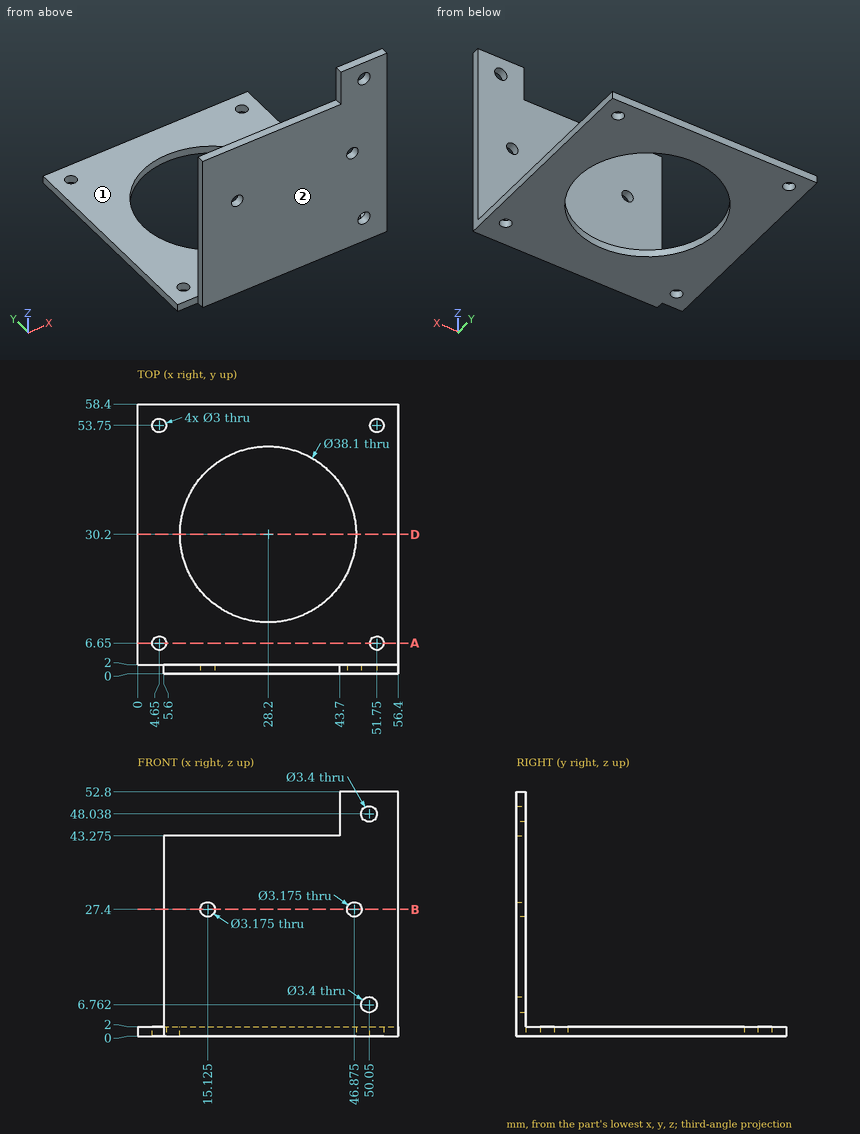
Geometry check sheet. Reference: drawing and pictorial views, mm from the part's lowest x, y, z. A direction names the side the tool comes from. Give positions to 0.01 mm unless a question says otherwise; leave off trailing zeros. Loops run counter-clockwise (first coordinate to the right, second up) from the corner with the lowest first, then second, coordinate; pieces in that order, holes last. Notation, with made-up numbers: M 55,-39.75 L 96,-39.75 A28 ccw 96,-15.75 Z; hole C 17,64 d8. An arc over 180 degrees is marked long. Use a Markdown table: item, result. Add a question column.
Q1. Sectioned sample at A-A, the plane y = 6.65. Record the cut outline in (x, z), then the cut area to 3 significant figures.
Q2. Tool access check on the marked faces 1 and 2. Record the directions out of +Z, -Z, +X, -X, +Y, -Y that give a thin tool (end or side, any length) a straight path to the whole face; none if there is none.
Q3. Scan lines: line 1 along X through (y, z) = (1.3, 27.4); line 2 along Y through (x, z) = (51.75, 0.4); line 3 along X through (y, z) = (30, 1). Record each from-to range of solid material in increasing order. Write a range as [from, to].
Q4. Sectioned sample at D-D, the plane y = 30.2. Record the cut outline in (x, z), then the cut area to 3 significant figures.
Q5. Sectioned sample at B-B, the plane z = 27.4. Record the cut outline in (x, y).
Q6. Go/stop test with flat-tipped pins: pin 1 (1.6 mm diameter, centred on x = 1.5, z = 1, fed in from -Y); pin 2 (1 mm diameter, centred on x = 27.5, y = 1, fed in from +Z) (1 decimal); pin 3 (2 mm diameter, centred on y = 1, z = 13, fed in from -X). Record where each tip stops, or that it passes through.
Verdict:
| question | item | result |
|---|---|---|
| 1 | outline | M 0,0 L 3.15,0 L 3.15,2 L 0,2 Z; M 6.15,0 L 50.25,0 L 50.25,2 L 6.15,2 Z; M 53.25,0 L 56.4,0 L 56.4,2 L 53.25,2 Z |
| 1 | area | 101 mm^2 |
| 2 | face 1 | +Z, +X, -X, +Y |
| 2 | face 2 | +Z, -Z, +X, -X, -Y |
| 3 | line 1 | [5.6, 13.54], [16.71, 45.29], [48.46, 56.4] |
| 3 | line 2 | [0, 5.15], [8.15, 52.25], [55.25, 58.4] |
| 3 | line 3 | [0, 9.15], [47.25, 56.4] |
| 4 | outline | M 0,0 L 9.15,0 L 9.15,2 L 0,2 Z; M 47.25,0 L 56.4,0 L 56.4,2 L 47.25,2 Z |
| 4 | area | 36.6 mm^2 |
| 5 | outline | M 5.6,0 L 13.54,0 L 13.54,2 L 5.6,2 Z; M 16.71,0 L 45.29,0 L 45.29,2 L 16.71,2 Z; M 48.46,0 L 56.4,0 L 56.4,2 L 48.46,2 Z |
| 6 | pin 1 | y = 2 |
| 6 | pin 2 | z = 43.3 |
| 6 | pin 3 | x = 5.6 |
